CAD build for the part. Positions are in the model's coordinates, mm. A direction names the side the tool comes from. Round coordinates to 2 decimals unless told otherwise and drop trailing zeros. Loops run counter-clockwise (first coordinate to the right, second up) from the corner with the lowest first, then second, coordinate; pieces in that order, holes last. Notation, with made-up numbers: (65, 15) -> (72, 15) arc R31 cw to (72, 45) -> close; hole circle Ø11 at (70.5, -4). An arc over 180 degrees is marked (long way). Answer as CSV lines item,"result".
```python
from build123d import *

# Parameters (mm, degrees)
SKETCH1_R           = 1
BOSS_EXTRUDE1_DEPTH = 3.4
BOSS_EXTRUDE3_DEPTH = 8.4
SKETCH5_R           = 1.2
BOSS_EXTRUDE6_DEPTH = 12.4
SKETCH6_R           = 0.65
CUT_EXTRUDE2_DEPTH  = 3
CUT_EXTRUDE3_START  = -2.34
CUT_EXTRUDE3_DEPTH  = 2.34
SKETCH8_R           = 1
CUT_EXTRUDE4_DEPTH  = 6


with BuildPart() as part:
    # Sketch1 → Boss-Extrude1 (new body)
    # profile 1 of 4: a face of its own
    with BuildSketch(Plane.XY):
        with BuildLine():
            Line((0, -2.625), (0, 2.625))
            Line((0, 2.625), (8.575, 2.625))
            ThreePointArc((8.575, 2.625), (9.724048519, 2.149048519), (10.2, 1))
            Line((10.2, 1), (10.2, -1))
            ThreePointArc((10.2, -1), (9.724048519, -2.149048519), (8.575, -2.625))
            Line((8.575, -2.625), (0, -2.625))
        make_face()
        Polygon((0.5, -2.125), (8.367893219, -2.125), (9.7, -0.792893219), (9.7, 0.792893219), (8.367893219, 2.125), (0.5, 2.125), align=None, mode=Mode.SUBTRACT)
    # profile 2 of 4: a face of its own
    with BuildSketch(Plane.XY):
        Polygon((0.5, -2.125), (0.5, 2.125), (8.367893219, 2.125), (9.7, 0.792893219), (9.7, -0.792893219), (8.367893219, -2.125), align=None)
        with Locations((2.6, 0)):
            Circle(SKETCH1_R, mode=Mode.SUBTRACT)
        with Locations((7.6, 0)):
            Circle(SKETCH1_R, mode=Mode.SUBTRACT)
    # profile 3 of 4: a face of its own
    with BuildSketch(Plane.XY):
        with Locations((7.6, 0)):
            Circle(SKETCH1_R)
    # profile 4 of 4: a face of its own
    with BuildSketch(Plane.XY):
        with Locations((2.6, 0)):
            Circle(SKETCH1_R)
    extrude(amount=BOSS_EXTRUDE1_DEPTH)

    # Sketch3 → Boss-Extrude3 (add)
    with BuildSketch(Plane(origin=(0, 0, 1), x_dir=(-1, 0, 0), z_dir=(0, 0, -1))):
        with BuildLine():
            Line((-5.613898291, -0.395), (-4.586101709, -0.395))
            ThreePointArc((-4.586101709, -0.395), (-3.884669218, -1.565327442), (-2.6, -2.025))
            Line((-2.6, -2.025), (-0.6, -2.025))
            Line((-0.6, -2.025), (-0.6, 2.025))
            Line((-0.6, 2.025), (-2.6, 2.025))
            ThreePointArc((-2.6, 2.025), (-3.884669218, 1.565327442), (-4.586101709, 0.395))
            Line((-4.586101709, 0.395), (-5.613898291, 0.395))
            ThreePointArc((-5.613898291, 0.395), (-6.315330782, 1.565327442), (-7.6, 2.025))
            Line((-7.6, 2.025), (-8.326471863, 2.025))
            Line((-8.326471863, 2.025), (-9.6, 0.751471863))
            Line((-9.6, 0.751471863), (-9.6, -0.751471863))
            Line((-9.6, -0.751471863), (-8.326471863, -2.025))
            Line((-8.326471863, -2.025), (-7.6, -2.025))
            ThreePointArc((-7.6, -2.025), (-6.315330782, -1.565327442), (-5.613898291, -0.395))
        make_face()
    extrude(amount=-BOSS_EXTRUDE3_DEPTH)

    # Sketch5 → Boss-Extrude6 (add)
    with BuildSketch(Plane.XY.offset(9.4)):
        with Locations((7.6, 0)):
            Circle(SKETCH5_R)
        with Locations((2.6, 0)):
            Circle(SKETCH5_R)
    extrude(amount=-BOSS_EXTRUDE6_DEPTH)

    # Sketch6 → Cut-Extrude2 (cut)
    with BuildSketch(Plane(origin=(0, 0, -3), x_dir=(-1, 0, 0), z_dir=(0, 0, -1))):
        with Locations((-7.6, 0)):
            Circle(SKETCH6_R)
        with Locations((-2.6, 0)):
            Circle(SKETCH6_R)
    extrude(amount=-CUT_EXTRUDE2_DEPTH, mode=Mode.SUBTRACT)

    # Sketch7 → Cut-Extrude3 (cut)
    with BuildSketch(Plane(origin=(0, 0, -3), x_dir=(-1, 0, 0), z_dir=(0, 0, -1)).offset(CUT_EXTRUDE3_START)):
        with BuildLine():
            Line((-2.6, -0.65), (-2.6, -1.2))
            ThreePointArc((-2.6, -1.2), (-1.751471863, -0.848528137), (-1.4, 0))
            ThreePointArc((-1.4, 0), (-1.751471863, 0.848528137), (-2.6, 1.2))
            Line((-2.6, 1.2), (-2.6, 0.65))
            ThreePointArc((-2.6, 0.65), (-2.140380592, 0.459619408), (-1.95, 0))
            ThreePointArc((-1.95, 0), (-2.140380592, -0.459619408), (-2.6, -0.65))
        make_face()
        with BuildLine():
            ThreePointArc((-7.6, 1.2), (-8.8, 0), (-7.6, -1.2))
            Line((-7.6, -1.2), (-7.6, 1.2))
        make_face()
    extrude(amount=CUT_EXTRUDE3_DEPTH, mode=Mode.SUBTRACT)

    # Sketch8 → Cut-Extrude4 (cut)
    with BuildSketch(Plane.XY.offset(9.4)):
        with Locations((7.6, 0)):
            Circle(SKETCH8_R)
        with Locations((2.6, 0)):
            Circle(SKETCH8_R)
    extrude(amount=-CUT_EXTRUDE4_DEPTH, mode=Mode.SUBTRACT)


solid = part.part
```
Q1. Slice it at D-D, the plane z = 0.25. Give the cut face in (x, y) (3 decimals).
Results:
outline,"(0, -2.625) -> (8.575, -2.625) arc R1.625 ccw to (10.2, -1) -> (10.2, 1) arc R1.625 ccw to (8.575, 2.625) -> (0, 2.625) -> close"
Q2. Probe L1, parallel to Y at x = 7.6, z = 5.1 (3 decimals); L2, parallel to X at y = -0.05, z = 4.75; L3, parallel to X at y = 0, z = -0.9. List the from-to ranges inside material, lowest first. Write a range as [from, to].
Results:
L1,"[-2.025, -1], [1, 2.025]"
L2,"[0.6, 1.6], [3.6, 6.6], [8.6, 9.6]"
L3,"[3.25, 3.8], [6.4, 6.95]"
Q3. Slice it at B-B, the plane x = 1. Give the cut face in (y, z) (3 decimals), and give its area (4 significant figures).
Results:
outline,"(-2.625, 0) -> (2.625, 0) -> (2.625, 3.4) -> (2.025, 3.4) -> (2.025, 9.4) -> (-2.025, 9.4) -> (-2.025, 3.4) -> (-2.625, 3.4) -> close"
area,"42.15 mm2"
Q4. Two-plate mould, pull along X, no slides. Class faces 6 (the flat face through (4, -2.625, 2)), 7 (the cylindrical face through (3.9, -1.553, 6.358)), 8 (the flat face through (0, 0, 2)), 9 (the cylindrical face through (6.4, 0.05, -1.15)): pulls with the +X half, pulls with the -X half, needs draft (parallel to the pull), parting line crosses it, or undercut.
Results:
face 6,"needs draft"
face 7,"undercut"
face 8,"pulls with the -X half"
face 9,"undercut"
Q5. Tool access for faces 1 (the cylindrical face through (6.8, -0.6, 6.4)), 2 (the flat face through (8.97, -1.38, 6.36)), 3 (the cylindrical face through (6.3, 1.553, 6.358)), 4 (the flat face through (2, 2.025, 6)), 5 (the flat face through (8.95, 1.4, 6.36)): list every direction of +Z, -Z, +X, -X, +Y, -Y with a clear straight run to the whole face (end or side of a thin tool).
Results:
face 1,"+Z"
face 2,"+Z, +X, -Y"
face 3,"+Z, +Y"
face 4,"+Z, +X, -X, +Y"
face 5,"+Z, +X, +Y"
Q6. Drop flat-ended pins along their axis: pin 1 Ø0.6 at (y, z) = (1, -2) entering from +X; pin 2 Ø2 at (x, z) = (2, 7) entering from +Y (3 decimals); pin 3 Ø0.8 at (x, y) = (2.6, 0) entering from -Z. Give the stop position or say it passes through.
Results:
pin 1,"x = 7.6"
pin 2,"y = 2.025"
pin 3,"z = 0"
Q7. Slice it at A-A, the plane z = 4. Give the cut face in (x, y) (3 decimals).
Results:
outline,"(0.6, -2.025) -> (2.6, -2.025) arc R2.025 ccw to (4.586, -0.395) -> (5.614, -0.395) arc R2.025 ccw to (7.6, -2.025) -> (8.326, -2.025) -> (9.6, -0.751) -> (9.6, 0.751) -> (8.326, 2.025) -> (7.6, 2.025) arc R2.025 ccw to (5.614, 0.395) -> (4.586, 0.395) arc R2.025 ccw to (2.6, 2.025) -> (0.6, 2.025) -> close; hole circle Ø2 at (2.6, 0); hole circle Ø2 at (7.6, 0)"
